Here's the drawing with two shaded views (mm, measured from the low corner). I have some questions. Coordinates: 2 decimals unless noted, no trailing zeros. Write each loop counter-clockwise with the first axis right and the second up, starting at its lowest first coordinate (ties: lowest second). Pieces come first, ordered by that corner, then holes.
Item 1: If we section it at B-B (y = 1.5): Please give me the cut outline in (x, z) (3 decimals), then the cut area to 3 significant figures.
Item 2: I'm going to push flat-ended pins straight in: pin 1 Ø6 at (x, z) = (10, 5) entering from -Y; pin 2 Ø1 at (y, z) = (2.5, 7.5) entering from +X; pin 3 Ø1.4 at (y, z) = (2.5, 7) entering from -X. Where does each tip first touch, or does it pass through?
Item 3: If we section it at C-C (x = 1): Please give me the cut outline in (y, z) (3 decimals).
Item 4: We'd pull the mould along X, two halves only. Please class the marked faces 1, 2 and 3: +X half, -X half, draft (parallel to the pull), parting line (faces both ways), or undercut.
Item 5: If we section it at D-D (z = 1.75): Please give me the cut outline in (x, y).
Item 6: If we section it at A-A (z = 6.73): Please give me the cut outline in (x, y) (3 decimals).
Item 7: If I drill on line 1 (X direction, y = 1, z = 6.73) (3 decimals); line 2 (X direction, y = 0.85, z = 1.65) (3 decimals); line 3 (Y direction, x = 1.75, z = 3), over which ranges is the centre line in solid material (lowest first)?
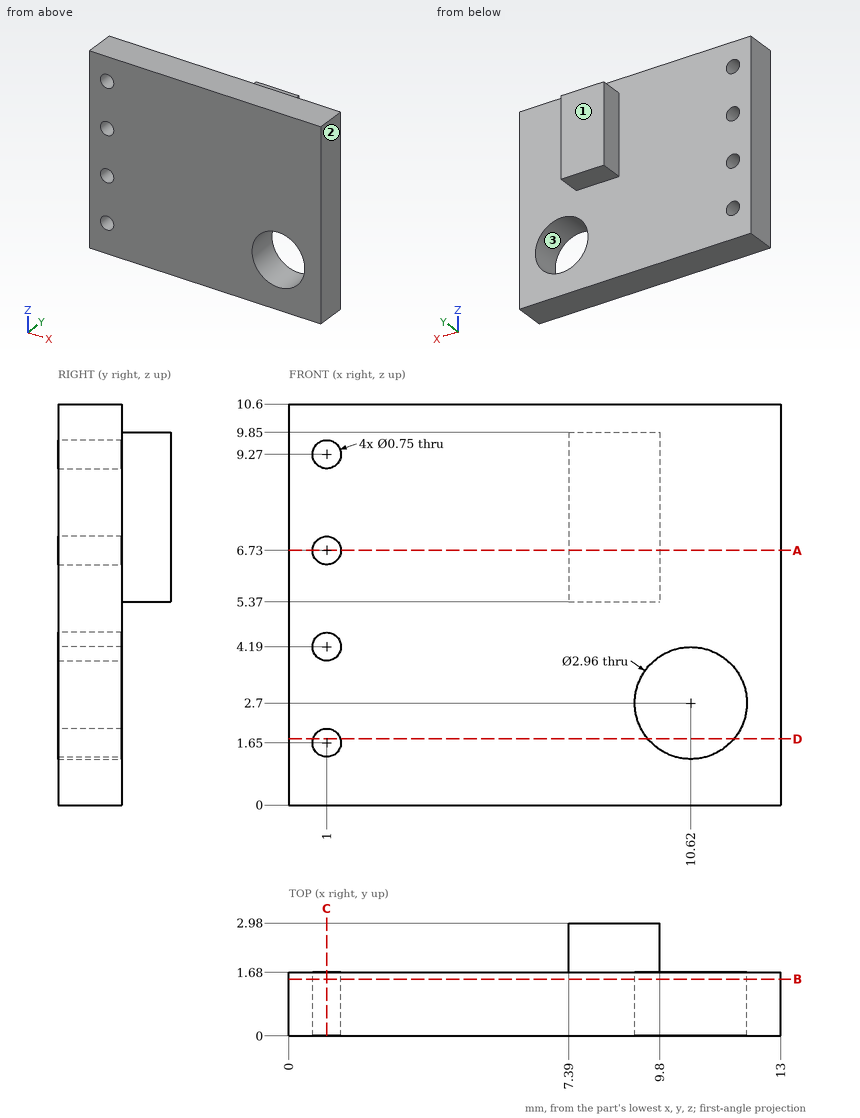
Answer list:
1. outline: (0, 0) - (13, 0) - (13, 10.6) - (0, 10.6) - close; hole circle Ø0.75 at (1, 1.65); hole circle Ø0.75 at (1, 4.19); hole circle Ø0.75 at (1, 6.73); hole circle Ø0.75 at (1, 9.27); hole circle Ø2.96 at (10.62, 2.7)
1. area: 129 mm2
2. pin 1: stops at y = 0
2. pin 2: stops at x = 9.8
2. pin 3: stops at x = 7.39
3. outline: (0, 0) - (1.68, 0) - (1.68, 1.275) - (0, 1.275) - close; (0, 2.025) - (1.68, 2.025) - (1.68, 3.815) - (0, 3.815) - close; (0, 4.565) - (1.68, 4.565) - (1.68, 6.355) - (0, 6.355) - close; (0, 7.105) - (1.68, 7.105) - (1.68, 8.895) - (0, 8.895) - close; (0, 9.645) - (1.68, 9.645) - (1.68, 10.6) - (0, 10.6) - close
4. face 1: draft
4. face 2: +X half
4. face 3: undercut
5. outline: (0, 0) - (0.64, 0) - (0.64, 1.68) - (0, 1.68) - close; (1.36, 0) - (9.49, 0) - (9.49, 1.68) - (1.36, 1.68) - close; (11.75, 0) - (13, 0) - (13, 1.68) - (11.75, 1.68) - close
6. outline: (0, 0) - (0.625, 0) - (0.625, 1.68) - (0, 1.68) - close; (1.375, 0) - (13, 0) - (13, 1.68) - (9.8, 1.68) - (9.8, 2.98) - (7.39, 2.98) - (7.39, 1.68) - (1.375, 1.68) - close
7. line 1: x = 0 to 0.625, 1.375 to 13
7. line 2: x = 0 to 0.625, 1.375 to 9.577, 11.663 to 13
7. line 3: y = 0 to 1.68
